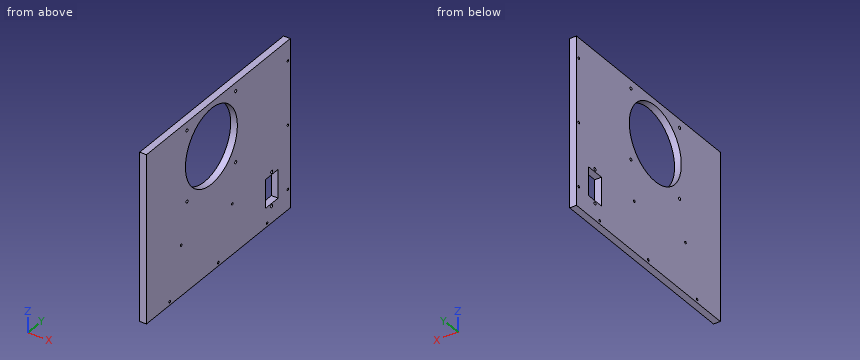
from build123d import *

# Parameters (mm, degrees)
CYLINDER033_R           = 1.7
CYLINDER033_DEPTH       = 20
CYLINDER031_R           = 1.7
CYLINDER031_DEPTH       = 20
CYLINDER031_ROLL_ANGLE  = 90
CYLINDER028_R           = 1.7
CYLINDER028_DEPTH       = 20
CYLINDER028_ROLL_ANGLE  = 90
CYLINDER032_R           = 1.7
CYLINDER032_DEPTH       = 20
CYLINDER030_R           = 1.7
CYLINDER030_DEPTH       = 20
CYLINDER030_ROLL_ANGLE  = 90
CYLINDER029_R           = 1.7
CYLINDER029_DEPTH       = 20
CYLINDER024_R           = 1.7
CYLINDER024_DEPTH       = 20
CYLINDER024_PITCH_ANGLE = 90
CYLINDER025_R           = 1.7
CYLINDER025_DEPTH       = 20
CYLINDER025_PITCH_ANGLE = 90
CYLINDER026_R           = 1.7
CYLINDER026_DEPTH       = 20
CYLINDER026_PITCH_ANGLE = 90
CYLINDER027_R           = 1.7
CYLINDER027_DEPTH       = 20
CYLINDER027_PITCH_ANGLE = 90
CYLINDER023_R           = 1.7
CYLINDER023_DEPTH       = 20
CYLINDER023_PITCH_ANGLE = 90
CYLINDER022_R           = 1.7
CYLINDER022_DEPTH       = 20
CYLINDER022_PITCH_ANGLE = 90
CYLINDER020_R           = 1.7
CYLINDER020_DEPTH       = 20
CYLINDER020_PITCH_ANGLE = 90
CYLINDER019_R           = 1.7
CYLINDER019_DEPTH       = 20
CYLINDER019_PITCH_ANGLE = 90
SKETCH018_R             = 2.2
SKETCH018_R_2           = 56
PAD016_DEPTH            = 20
SKETCH012_R             = 2.2
SKETCH012_W             = 27.8
SKETCH012_H             = 42.5
PAD012_DEPTH            = 30
SKETCH006_W             = 310
SKETCH006_H             = 250
PAD006_DEPTH            = 10


with BuildPart() as cylinder033:
    # Cylinder033 → Cylinder033 (new body)
    with BuildSketch(Plane(origin=(-205, 120, 240), x_dir=(1, 0, 0), z_dir=(0, 0, 1))):
        Circle(CYLINDER033_R)
    extrude(amount=CYLINDER033_DEPTH)


with BuildPart() as cylinder031:
    # Cylinder031 → Cylinder031 (new body)
    with BuildSketch(Plane.XY):
        Circle(CYLINDER031_R)
    extrude(amount=CYLINDER031_DEPTH)


with BuildPart() as cylinder031_1:
    # Cylinder031 roll: moved
    add(cylinder031.part.rotate(Axis((0, 0, 0), (1, 0, 0)), CYLINDER031_ROLL_ANGLE))


with BuildPart() as cylinder031_2:
    # Cylinder031 placement: moved
    add(cylinder031_1.part.moved(Location((-205, -140, 210))))


with BuildPart() as cylinder028:
    # Cylinder028 → Cylinder028 (new body)
    with BuildSketch(Plane.XY):
        Circle(CYLINDER028_R)
    extrude(amount=CYLINDER028_DEPTH)


with BuildPart() as cylinder028_1:
    # Cylinder028 roll: moved
    add(cylinder028.part.rotate(Axis((0, 0, 0), (1, 0, 0)), CYLINDER028_ROLL_ANGLE))


with BuildPart() as cylinder028_2:
    # Cylinder028 placement: moved
    add(cylinder028_1.part.moved(Location((-205, -140, 20))))


with BuildPart() as cylinder032:
    # Cylinder032 → Cylinder032 (new body)
    with BuildSketch(Plane(origin=(-205, 15, 240), x_dir=(1, 0, 0), z_dir=(0, 0, 1))):
        Circle(CYLINDER032_R)
    extrude(amount=CYLINDER032_DEPTH)


with BuildPart() as cylinder030:
    # Cylinder030 → Cylinder030 (new body)
    with BuildSketch(Plane.XY):
        Circle(CYLINDER030_R)
    extrude(amount=CYLINDER030_DEPTH)


with BuildPart() as cylinder030_1:
    # Cylinder030 roll: moved
    add(cylinder030.part.rotate(Axis((0, 0, 0), (1, 0, 0)), CYLINDER030_ROLL_ANGLE))


with BuildPart() as cylinder030_2:
    # Cylinder030 placement: moved
    add(cylinder030_1.part.moved(Location((-205, -140, 115))))


with BuildPart() as fusion006:
    # Cylinder029 → Cylinder029 (new body)
    with BuildSketch(Plane(origin=(-205, -90, 240), x_dir=(1, 0, 0), z_dir=(0, 0, 1))):
        Circle(CYLINDER029_R)
    extrude(amount=CYLINDER029_DEPTH)

    # Fusion006: union Cylinder033, Cylinder031, Cylinder028, Cylinder032, Cylinder030
    add(cylinder033.part)
    add(cylinder031_2.part)
    add(cylinder028_2.part)
    add(cylinder032.part)
    add(cylinder030_2.part)


with BuildPart() as cylinder024:
    # Cylinder024 → Cylinder024 (new body)
    with BuildSketch(Plane.XY):
        Circle(CYLINDER024_R)
    extrude(amount=CYLINDER024_DEPTH)


with BuildPart() as cylinder024_1:
    # Cylinder024 pitch: moved
    add(cylinder024.part.rotate(Axis((0, 0, 0), (0, 1, 0)), CYLINDER024_PITCH_ANGLE))


with BuildPart() as cylinder024_2:
    # Cylinder024 placement: moved
    add(cylinder024_1.part.moved(Location((-220, 120, -5))))


with BuildPart() as cylinder025:
    # Cylinder025 → Cylinder025 (new body)
    with BuildSketch(Plane.XY):
        Circle(CYLINDER025_R)
    extrude(amount=CYLINDER025_DEPTH)


with BuildPart() as cylinder025_1:
    # Cylinder025 pitch: moved
    add(cylinder025.part.rotate(Axis((0, 0, 0), (0, 1, 0)), CYLINDER025_PITCH_ANGLE))


with BuildPart() as cylinder025_2:
    # Cylinder025 placement: moved
    add(cylinder025_1.part.moved(Location((-220, 165, 20))))


with BuildPart() as cylinder026:
    # Cylinder026 → Cylinder026 (new body)
    with BuildSketch(Plane.XY):
        Circle(CYLINDER026_R)
    extrude(amount=CYLINDER026_DEPTH)


with BuildPart() as cylinder026_1:
    # Cylinder026 pitch: moved
    add(cylinder026.part.rotate(Axis((0, 0, 0), (0, 1, 0)), CYLINDER026_PITCH_ANGLE))


with BuildPart() as cylinder026_2:
    # Cylinder026 placement: moved
    add(cylinder026_1.part.moved(Location((-220, 165, 115))))


with BuildPart() as cylinder027:
    # Cylinder027 → Cylinder027 (new body)
    with BuildSketch(Plane.XY):
        Circle(CYLINDER027_R)
    extrude(amount=CYLINDER027_DEPTH)


with BuildPart() as cylinder027_1:
    # Cylinder027 pitch: moved
    add(cylinder027.part.rotate(Axis((0, 0, 0), (0, 1, 0)), CYLINDER027_PITCH_ANGLE))


with BuildPart() as cylinder027_2:
    # Cylinder027 placement: moved
    add(cylinder027_1.part.moved(Location((-220, 165, 210))))


with BuildPart() as cylinder023:
    # Cylinder023 → Cylinder023 (new body)
    with BuildSketch(Plane.XY):
        Circle(CYLINDER023_R)
    extrude(amount=CYLINDER023_DEPTH)


with BuildPart() as cylinder023_1:
    # Cylinder023 pitch: moved
    add(cylinder023.part.rotate(Axis((0, 0, 0), (0, 1, 0)), CYLINDER023_PITCH_ANGLE))


with BuildPart() as cylinder023_2:
    # Cylinder023 placement: moved
    add(cylinder023_1.part.moved(Location((-220, 15, -5))))


with BuildPart() as fusion007:
    # Cylinder022 → Cylinder022 (new body)
    with BuildSketch(Plane.XY):
        Circle(CYLINDER022_R)
    extrude(amount=CYLINDER022_DEPTH)


with BuildPart() as fusion007_1:
    # Cylinder022 pitch: moved
    add(fusion007.part.rotate(Axis((0, 0, 0), (0, 1, 0)), CYLINDER022_PITCH_ANGLE))


with BuildPart() as fusion007_2:
    # Cylinder022 placement: moved
    add(fusion007_1.part.moved(Location((-220, -90, -5))))

    # Fusion007: union Cylinder024, Cylinder025, Cylinder026, Cylinder027, Cylinder023
    add(cylinder024_2.part)
    add(cylinder025_2.part)
    add(cylinder026_2.part)
    add(cylinder027_2.part)
    add(cylinder023_2.part)


with BuildPart() as cylinder020:
    # Cylinder020 → Cylinder020 (new body)
    with BuildSketch(Plane.XY):
        Circle(CYLINDER020_R)
    extrude(amount=CYLINDER020_DEPTH)


with BuildPart() as cylinder020_1:
    # Cylinder020 pitch: moved
    add(cylinder020.part.rotate(Axis((0, 0, 0), (0, 1, 0)), CYLINDER020_PITCH_ANGLE))


with BuildPart() as cylinder020_2:
    # Cylinder020 placement: moved
    add(cylinder020_1.part.moved(Location((-220, 45, 65))))


with BuildPart() as fusion009:
    # Cylinder019 → Cylinder019 (new body)
    with BuildSketch(Plane.XY):
        Circle(CYLINDER019_R)
    extrude(amount=CYLINDER019_DEPTH)


with BuildPart() as fusion009_1:
    # Cylinder019 pitch: moved
    add(fusion009.part.rotate(Axis((0, 0, 0), (0, 1, 0)), CYLINDER019_PITCH_ANGLE))


with BuildPart() as fusion009_2:
    # Cylinder019 placement: moved
    add(fusion009_1.part.moved(Location((-220, -65, 65))))

    # Fusion008: union Cylinder020
    add(cylinder020_2.part)

    # Fusion009: union Fusion006, Fusion007
    add(fusion006.part)
    add(fusion007_2.part)


with BuildPart() as pad016:
    # Sketch018 → Pad016 (new body)
    with BuildSketch(Plane(origin=(-200, 0, 175), x_dir=(0, 1, 0), z_dir=(1, 0, 0))):
        with Locations((-52.5, 52.5)):
            Circle(SKETCH018_R)
        with Locations((52.5, 52.5)):
            Circle(SKETCH018_R)
        with Locations((-52.5, -52.5)):
            Circle(SKETCH018_R)
        with Locations((52.5, -52.5)):
            Circle(SKETCH018_R)
        Circle(SKETCH018_R_2)
    extrude(amount=-PAD016_DEPTH)


with BuildPart() as pad012:
    # Sketch012 → Pad012 (new body)
    with BuildSketch(Plane(origin=(-213, 130, 40), x_dir=(0, 1, 0), z_dir=(1, 0, 0))):
        with Locations((0, 25.3)):
            Circle(SKETCH012_R)
        with Locations((0, -25.3)):
            Circle(SKETCH012_R)
        Rectangle(SKETCH012_W, SKETCH012_H)
    extrude(amount=PAD012_DEPTH)


with BuildPart() as cut012:
    # Sketch006 → Pad006 (new body)
    with BuildSketch(Plane.YZ.offset(-210)):
        with Locations((15, 115)):
            Rectangle(SKETCH006_W, SKETCH006_H)
    extrude(amount=PAD006_DEPTH)

    # Cut004: cut Pad012
    add(pad012.part, mode=Mode.SUBTRACT)

    # Cut011: cut Pad016
    add(pad016.part, mode=Mode.SUBTRACT)

    # Cut012: cut Fusion009
    add(fusion009_2.part, mode=Mode.SUBTRACT)


solid = cut012.part
Check sheet for the modelled part. Datum: model origin and axes. Units: mm. Round coordinates to 2 decimals unless told otherwise and drop trailing zeros. Write each loop counter-clockwise with the first axis right and the second up, starting at its lowest first coordinate (ties: lowest second). Pieces come first, ordered by that corner, then holes. Notation, with made-up numbers: (38, 12) -> (97, 12) arc R29 ccw to (97, 51) -> close; hole circle Ø5 at (-11, 28.25). An arc over 180 degrees is marked (long way). Answer as CSV lines item,"result". Start each with the question number.
1) Section check B-B on x = -208.5. State how many separate pieces and enclosed holes the cut face has, and give its area (3 significant figures).
2) Material ranges on line 1 (Y direction, x = -203.25, z = 65); line 2 (Y direction, x = -202.5, z = 20); line 3 (Z direction, x = -204.5, y = 15), recorded low to high. Write a range as from..to.
3) Section check A-A on z = 50. Enter the section's corners in (x, y).
4) Section check C-C on z = 175. Enter the section's corners in (x, y).
5) Go/stop test with a flat-tipped pin: P1, Ø2.5, axis at y = -65, z = 65, coming from the -X side. Record where the tip stops, or that it passes through.
Found:
1,separate pieces,"1"
1,enclosed holes,"16"
1,area,"66,300 mm^2"
2,line 1,"y = -140..-66.7, -63.3..43.3, 46.7..127.82, 132.18..170"
2,line 2,"y = -140..116.1, 143.9..163.3, 166.7..170"
2,line 3,"z = -10..-6.7, -3.3..121.05, 228.95..240"
3,outline,"(-210, -140) -> (-200, -140) -> (-200, 116.1) -> (-210, 116.1) -> close; (-210, 143.9) -> (-200, 143.9) -> (-200, 170) -> (-210, 170) -> close"
4,outline,"(-210, -140) -> (-200, -140) -> (-200, -56) -> (-210, -56) -> close; (-210, 56) -> (-200, 56) -> (-200, 170) -> (-210, 170) -> close"
5,P1,"passes through"
